Geometry check sheet. Reference: the model listing, model coordinates, mm. A direction names the side the tool comes from. Round coordinates to 2 decimals unless told otherwise and drop trailing zeros. Write each loop counter-clockwise with the first axis right and the second up, starting at its lowest first coordinate (ties: lowest second). Pieces come first, ordered by that corner, then holes. Notation, with made-up numbers: M -9,-3 L 27,-3 A34 ccw 27,27 Z; hole C 43,6.5 d5. An arc over 180 degrees is marked long. Put each result on its own line as item: value. Start each with the question number.
(1) Section check B-B on z = 1.4. Count the separate pieces of the cut face and the enclosed holes in it, then the cut area to 3 significant figures.
(2) Gauge pin test, flat ends, axial feed: pin 1 (1.1 mm diameter, centred on x = -76, z = 0.5, fed in from +Y); pin 2 (5 mm diameter, centred on x = -68.76, y = 10.5, fed in from +Z); pin 3 (2.5 mm diameter, centred on x = -53.5, y = 32, fed in from +Z). Record the tip position at first contact, or that the pin passes through.
(3) Mould release check, pull along Y, two halves, no side actions. Record for faces 4 (the cylindrical face through (-81.55, 14.39, 1.49)), 5 (the flat face through (-96, 5.5, 0.5)), 6 (the cylindrical face through (-90, 6, 1.5)): pulls with the +Y half, pulls with the -Y half, needs draft (parallel to the pull), parting line crosses it, or undercut.
(4) Section check C-C on x = -53. Record the cut outline in (y, z), then the cut area to 3 significant figures.
(5) Material ranges on probe 1 along Y at (x, z) = (-53.5, 0.4); probe 2 along X at (y, z) = (11, 0.55); probe 3 along Y at (x, z) = (-91, 0.3), recorded low to high.
(6) Section check A-A on x = -89. Record the cut outline in (y, z).
(7) Tool access check on faces 1 (the flat face through (-45, 6, 2)), 2 (the cylindrical face through (-70, 6, 1.5)), 3 (the cylindrical face through (-45.57, 11.6, 1.49)). Record the directions out of +Z, -Z, +X, -X, +Y, -Y that give a thin tool (end or side, any length) a straight path to the whole face; none if there is none.
(8) Section check D-D on y = 20. Record the cut outline in (x, z), then the cut area to 3 significant figures.
from build123d import *

# Parameters (mm, degrees)
BOSS_EXTRUDE1_DEPTH = 1
SKETCH2_R           = 1
BOSS_EXTRUDE2_DEPTH = 1
FILLET1_R           = 3
CUT_EXTRUDE1_REACH  = 3
SKETCH3_R           = 1.55


with BuildPart() as part:
    # Sketch1 → Boss-Extrude1 (new body)
    with BuildSketch(Plane.XY):
        Polygon((-96, 3), (-41, 3), (-41, 38), (-66, 38), (-66, 18), (-86, 18), (-96, 8), align=None)
    extrude(amount=BOSS_EXTRUDE1_DEPTH)

    # Sketch2 → Boss-Extrude2 (add)
    with BuildSketch(Plane.XY.offset(1)):
        with BuildLine():
            Line((-47, 11), (-60, 11))
            ThreePointArc((-60, 11), (-61.414213562, 11.585786438), (-62, 13))
            Line((-62, 13), (-62, 21))
            ThreePointArc((-62, 21), (-61.414213562, 22.414213562), (-60, 23))
            Line((-60, 23), (-47, 23))
            ThreePointArc((-47, 23), (-45.585786438, 22.414213562), (-45, 21))
            Line((-45, 21), (-45, 13))
            ThreePointArc((-45, 13), (-45.585786438, 11.585786438), (-47, 11))
        make_face()
        with Locations((-63, 26)):
            Circle(SKETCH2_R)
        with Locations((-63, 29)):
            Circle(SKETCH2_R)
        with Locations((-63, 32)):
            Circle(SKETCH2_R)
        with Locations((-63, 35)):
            Circle(SKETCH2_R)
        with Locations((-60, 35)):
            Circle(SKETCH2_R)
        with Locations((-57, 35)):
            Circle(SKETCH2_R)
        with Locations((-50, 35)):
            Circle(SKETCH2_R)
        with Locations((-47, 35)):
            Circle(SKETCH2_R)
        with Locations((-44, 32)):
            Circle(SKETCH2_R)
        with Locations((-44, 29)):
            Circle(SKETCH2_R)
        with Locations((-44, 26)):
            Circle(SKETCH2_R)
        with Locations((-45, 6)):
            Circle(SKETCH2_R)
        with Locations((-49, 6)):
            Circle(SKETCH2_R)
        with Locations((-53, 6)):
            Circle(SKETCH2_R)
        with Locations((-57, 6)):
            Circle(SKETCH2_R)
        with Locations((-61, 6)):
            Circle(SKETCH2_R)
        with Locations((-65, 6)):
            Circle(SKETCH2_R)
        with Locations((-69, 6)):
            Circle(SKETCH2_R)
        with Locations((-73, 6)):
            Circle(SKETCH2_R)
        with Locations((-77, 6)):
            Circle(SKETCH2_R)
        with Locations((-81, 6)):
            Circle(SKETCH2_R)
        with Locations((-85, 6)):
            Circle(SKETCH2_R)
        with Locations((-89, 6)):
            Circle(SKETCH2_R)
        with Locations((-93, 6)):
            Circle(SKETCH2_R)
        with Locations((-84.757359313, 15)):
            Circle(SKETCH2_R)
        with Locations((-76.757359313, 15)):
            Circle(SKETCH2_R)
        with Locations((-72.757359313, 15)):
            Circle(SKETCH2_R)
        with Locations((-68.757359313, 15)):
            Circle(SKETCH2_R)
        with Locations((-64.757359313, 15)):
            Circle(SKETCH2_R)
        with Locations((-44, 35)):
            Circle(SKETCH2_R)
        with Locations((-80.757359313, 15)):
            Circle(SKETCH2_R)
    extrude(amount=BOSS_EXTRUDE2_DEPTH)

    # Fillet1
    fillet1_edges = [part.edges().sort_by_distance(p)[0] for p in [
        (-41, 38, 0.5),
        (-41, 3, 0.5),
        (-86, 18, 0.5),
        (-66, 18, 0.5),
        (-66, 38, 0.5),
    ]]
    fillet(fillet1_edges, radius=FILLET1_R)

    # Sketch3 → Cut-Extrude1 (cut, up to next)
    with BuildSketch(Plane.XY.offset(1), mode=Mode.PRIVATE) as cut_extrude1_sk1:
        with Locations((-53.5, 32)):
            Circle(SKETCH3_R)
    cut_extrude1_tool1 = extrude(cut_extrude1_sk1.sketch, amount=-CUT_EXTRUDE1_REACH, mode=Mode.PRIVATE) & part.part
    add(cut_extrude1_tool1.solids().sort_by_distance((-53.5, 32, 1))[0], mode=Mode.SUBTRACT)
    # Sketch3 → Cut-Extrude1 (cut, up to next)
    with BuildSketch(Plane.XY.offset(1), mode=Mode.PRIVATE) as cut_extrude1_sk2:
        with Locations((-68.757359313, 10.5)):
            Circle(SKETCH3_R)
    cut_extrude1_tool2 = extrude(cut_extrude1_sk2.sketch, amount=-CUT_EXTRUDE1_REACH, mode=Mode.PRIVATE) & part.part
    add(cut_extrude1_tool2.solids().sort_by_distance((-68.757359, 10.5, 1))[0], mode=Mode.SUBTRACT)
    # Sketch3 → Cut-Extrude1 (cut, up to next)
    with BuildSketch(Plane.XY.offset(1), mode=Mode.PRIVATE) as cut_extrude1_sk3:
        with Locations((-80.757359313, 10.5)):
            Circle(SKETCH3_R)
    cut_extrude1_tool3 = extrude(cut_extrude1_sk3.sketch, amount=-CUT_EXTRUDE1_REACH, mode=Mode.PRIVATE) & part.part
    add(cut_extrude1_tool3.solids().sort_by_distance((-80.757359, 10.5, 1))[0], mode=Mode.SUBTRACT)


solid = part.part
Answers follow:
1. separate pieces: 32
1. enclosed holes: 0
1. area: 298 mm^2
2. pin 1: stops at y = 18
2. pin 2: stops at z = 1
2. pin 3: passes through
3. face 4: undercut
3. face 5: needs draft
3. face 6: parting line crosses it
4. outline: M 3,0 L 30.53,0 L 30.53,1 L 23,1 L 23,2 L 11,2 L 11,1 L 7,1 L 7,2 L 5,2 L 5,1 L 3,1 Z; M 33.47,0 L 38,0 L 38,1 L 33.47,1 Z
4. area: 46.1 mm^2
5. probe 1: y = 3 to 30.45, 33.55 to 38
5. probe 2: x = -93 to -82.22, -79.29 to -70.22, -67.29 to -41
5. probe 3: y = 3 to 13
6. outline: M 3,0 L 15,0 L 15,1 L 7,1 L 7,2 L 5,2 L 5,1 L 3,1 Z
7. face 1: +Z, +X, -X, +Y, -Y
7. face 2: +Z
7. face 3: +Z, +X
8. outline: M -66.17,0 L -41,0 L -41,1 L -45,1 L -45,2 L -62,2 L -62,1 L -66.17,1 Z
8. area: 42.2 mm^2
